from build123d import *

# Parameters (mm, degrees)
SKETCH_2_W          = 95.3
SKETCH_2_H          = 120
EXTRUDE_2_DEPTH     = 1.6
SKETCH_3_R          = 1.8
SKETCH_3_W          = 4
SKETCH_3_H          = 7
SKETCH_3_W_2        = 6
SKETCH_3_H_2        = 4
CUT_EXTRUDE_1_DEPTH = 2.6


with BuildPart() as part:
    # 스케치2 → 보스-돌출2 (new body)
    with BuildSketch(Plane.XY):
        Rectangle(SKETCH_2_W, SKETCH_2_H)
    extrude(amount=EXTRUDE_2_DEPTH)

    # 스케치3 → 컷-돌출1 (cut, through all)
    with BuildSketch(Plane.XY.offset(1.6)):
        with Locations((-38.35, 52)):
            Circle(SKETCH_3_R)
        with Locations((41.65, 52)):
            Circle(SKETCH_3_R)
        with Locations((41.65, -56)):
            Circle(SKETCH_3_R)
        with Locations((-43.35, -53)):
            Circle(SKETCH_3_R)
        with Locations((-45.65, 56.5)):
            Rectangle(SKETCH_3_W, SKETCH_3_H)
        with Locations((-44.65, -58)):
            Rectangle(SKETCH_3_W_2, SKETCH_3_H_2)
    extrude(amount=-CUT_EXTRUDE_1_DEPTH, mode=Mode.SUBTRACT)


solid = part.part
Can you work these out from the model? Positions are in its coordinate system, mm. Round coordinates to 2 decimals unless told otherwise and drop trailing zeros. Write each question's results on one line, items separated by ' | '. Start each with the question number.
Item 1: Will these pins go through, and if not, where does the flat tip stop? pin 1 (0.5 mm diameter, centred on x = -44, z = 0.5, fed in from -Y); pin 2 (0.5 mm diameter, centred on y = -57, z = 0.5, fed in from -X).
Item 2: Please list where these lines run through material, in increasing order: L1, parallel to Y at x = 41.65, z = 0.55; L2, parallel to Y at x = -38.35, z = 0.5; L3, parallel to Y at x = -43.35, z = 0.8.
Item 3: Thinking about a two-plate mould opening in X: for faces 1 (the cylindrical face through (-42.382, -51.482, 0.811)), 2 (the flat face through (-1, 1, 1.6)), which applies, +X half, -X half, draft (parallel to the pull), parting line (faces both ways), or undercut?
Results:
1) pin 1: stops at y = -56 | pin 2: stops at x = -41.65
2) L1: y = -60 to -57.8, -54.2 to 50.2, 53.8 to 60 | L2: y = -60 to 50.2, 53.8 to 60 | L3: y = -56 to -54.8, -51.2 to 60
3) face 1: undercut | face 2: draft
